Here's how the part is built. I have some questions about the finished solid (model axes, mm). Face numbers are marked on the shaded views. A direction names the side the tool comes from. Round coordinates to 2 decimals unless told otherwise and drop trailing zeros. Write each loop counter-clockwise with the first axis right and the second up, starting at its lowest first coordinate (ties: lowest second). Pieces come first, ordered by that corner, then holes. Notation, with made-up numbers: M 18,70.25 L 47,70.25 A34 ccw 47,105.25 Z; hole C 37.5,20 d11. An arc over 180 degrees is marked long. Use one line per item in the form item = value. Start each with the question number.
Q1. I want a section at D-D on x = -4.25. List the corners of the cut face in (y, z) for me, and give its area (3 significant figures).
Q2. I need wall thicknesses on line 1 along X through (y, z) = (-0.5, 10.75); line 2 along X through (y, z) = (3, 7.5); line 3 along Z through (x, y) = (-3.75, 10). Which ranges of each line are inside material? Lowest first, please. Write a range as from..to.
Q3. For the marked faces 1, 2 and 3, which set-ups out of +Z, -Z, +X, -X, +Y, -Y let a thin tool reach every point of the face, with its end or its side?
Q4. I want a section at B-B on z = 12.75. List the corners of the cut face in (x, y) for me.
Q5. I want a section at A-A on y = -1.5. List the corners of the cut face in (x, z) for me.
Q6. We'd pull the mould along Z, two halves only. Please class the marked faces 4, 5, 6 and 7: +Z half, -Z half, draft (parallel to the pull), parting line (faces both ways), or undercut.
Q7. I'm going to push flat-ended pins straight in: pin 1 Ø1.5 at (x, y) = (2, 10.5) entering from +Z; pin 2 Ø5.5 at (x, z) = (0, 7.5) entering from -Y; pin 3 Ø5.5 at (x, z) = (-2.5, 2.5) entering from +Y. Where does each tip first touch, or does it pass through?
Q8. I want a section at C-C on x = 0. List the corners of the cut face in (y, z) for me.
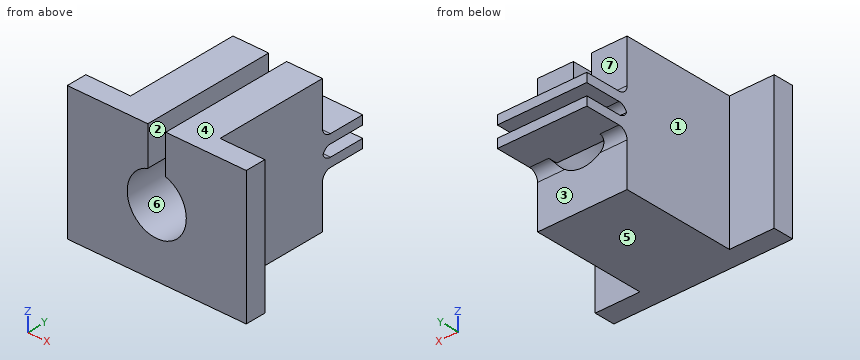
```python
from build123d import *

# Parameters (mm, degrees)
SKETCH1_W           = 10
SKETCH1_H           = 15
BOSS_EXTRUDE1_DEPTH = 15
SKETCH3_W           = 5
SKETCH3_H           = 2.3
BOSS_EXTRUDE2_DEPTH = 15
SKETCH4_R           = 3.3
CUT_EXTRUDE1_DEPTH  = 24.452078799
SKETCH6_W           = 2
SKETCH6_H           = 15
CUT_EXTRUDE2_DEPTH  = 8
SKETCH7_W           = 10
SKETCH7_H           = 1
BOSS_EXTRUDE3_DEPTH = 5
FILLET1_R           = 1


with BuildPart() as part:
    # Sketch1 → Boss-Extrude1 (new body)
    with BuildSketch(Plane.XY):
        Rectangle(SKETCH1_W, SKETCH1_H)
    extrude(amount=BOSS_EXTRUDE1_DEPTH)

    # Sketch3 → Boss-Extrude2 (add)
    with BuildSketch(Plane.XY.offset(15)):
        with Locations((-7.5, -6.35)):
            Rectangle(SKETCH3_W, SKETCH3_H)
        with Locations((7.5, -6.35)):
            Rectangle(SKETCH3_W, SKETCH3_H)
    extrude(amount=-BOSS_EXTRUDE2_DEPTH)

    # Sketch4 → Cut-Extrude1 (cut, through all)
    with BuildSketch(Plane.XZ.offset(7.5)):
        with Locations(Location((0, 7.5, 0), (0, 0, 270))):
            Circle(SKETCH4_R)
    extrude(amount=-CUT_EXTRUDE1_DEPTH, mode=Mode.SUBTRACT)

    # Sketch6 → Cut-Extrude2 (cut)
    with BuildSketch(Plane.XY.offset(15)):
        Rectangle(SKETCH6_W, SKETCH6_H)
    extrude(amount=-CUT_EXTRUDE2_DEPTH, mode=Mode.SUBTRACT)

    # Sketch7 → Boss-Extrude3 (add)
    with BuildSketch(Plane(origin=(0, 7.5, 0), x_dir=(1, 0, 0), z_dir=(0, 1, 0))):
        with Locations((0, -8.65)):
            Rectangle(SKETCH7_W, SKETCH7_H)
        with Locations((0, -6.35)):
            Rectangle(SKETCH7_W, SKETCH7_H)
    extrude(amount=BOSS_EXTRUDE3_DEPTH)

    # Fillet1
    # the kernel refuses this fillet: 1 mm, written as the material it adds along each edge
    with BuildSketch(Plane(origin=(5, 7.5, 5.85), x_dir=(0, 0, -1), z_dir=(-1, 0, 0))) as fillet1_piece_1_section:
        with BuildLine():
            CenterArc((FILLET1_R, -FILLET1_R), FILLET1_R, 90, 90)
            Line((0, -FILLET1_R), (0, 0))
            Line((0, 0), (FILLET1_R, 0))
        make_face()
    fillet1_piece_1 = extrude(amount=4.642116168, mode=Mode.PRIVATE)
    fillet1_piece_1 = fillet1_piece_1 - Plane(origin=(0, 7.716795794, 7.5), x_dir=(0, 0, -1), z_dir=(0, -1, 0)) * Cylinder(3.3, 14, mode=Mode.PRIVATE)
    add(fillet1_piece_1)
    with BuildSketch(Plane(origin=(0.735351604, 7.5, 6.85), x_dir=(0, 0, 1), z_dir=(1, 0, 0))) as fillet1_piece_2_section:
        with BuildLine():
            CenterArc((FILLET1_R, -FILLET1_R), FILLET1_R, 90, 90)
            Line((0, -FILLET1_R), (0, 0))
            Line((0, 0), (FILLET1_R, 0))
        make_face()
    fillet1_piece_2 = extrude(amount=4.264648396, mode=Mode.PRIVATE)
    fillet1_piece_2 = fillet1_piece_2 - Plane(origin=(0, 7.724716743, 7.5), x_dir=(0, 0, -1), z_dir=(0, -1, 0)) * Cylinder(3.3, 13, mode=Mode.PRIVATE)
    add(fillet1_piece_2)
    with BuildSketch(Plane(origin=(-0.357883832, 7.5, 5.85), x_dir=(0, 0, -1), z_dir=(-1, 0, 0))) as fillet1_piece_3_section:
        with BuildLine():
            CenterArc((FILLET1_R, -FILLET1_R), FILLET1_R, 90, 90)
            Line((0, -FILLET1_R), (0, 0))
            Line((0, 0), (FILLET1_R, 0))
        make_face()
    fillet1_piece_3 = extrude(amount=4.642116168, mode=Mode.PRIVATE)
    fillet1_piece_3 = fillet1_piece_3 - Plane(origin=(0, 7.716795859, 7.5), x_dir=(0, 0, -1), z_dir=(0, -1, 0)) * Cylinder(3.3, 14, mode=Mode.PRIVATE)
    add(fillet1_piece_3)
    with BuildSketch(Plane(origin=(-5, 7.5, 6.85), x_dir=(0, 0, 1), z_dir=(1, 0, 0))) as fillet1_piece_4_section:
        with BuildLine():
            CenterArc((FILLET1_R, -FILLET1_R), FILLET1_R, 90, 90)
            Line((0, -FILLET1_R), (0, 0))
            Line((0, 0), (FILLET1_R, 0))
        make_face()
    fillet1_piece_4 = extrude(amount=4.264648396, mode=Mode.PRIVATE)
    fillet1_piece_4 = fillet1_piece_4 - Plane(origin=(0, 7.724717828, 7.5), x_dir=(0, 0, -1), z_dir=(0, -1, 0)) * Cylinder(3.3, 13, mode=Mode.PRIVATE)
    add(fillet1_piece_4)
    with BuildSketch(Plane(origin=(-0.735351604, 7.5, 8.15), x_dir=(0, 0, -1), z_dir=(-1, 0, 0))) as fillet1_piece_5_section:
        with BuildLine():
            CenterArc((FILLET1_R, -FILLET1_R), FILLET1_R, 90, 90)
            Line((0, -FILLET1_R), (0, 0))
            Line((0, 0), (FILLET1_R, 0))
        make_face()
    fillet1_piece_5 = extrude(amount=4.264648396, mode=Mode.PRIVATE)
    fillet1_piece_5 = fillet1_piece_5 - Plane(origin=(0, 7.724716743, 7.5), x_dir=(0, 0, -1), z_dir=(0, -1, 0)) * Cylinder(3.3, 13, mode=Mode.PRIVATE)
    add(fillet1_piece_5)
    with BuildSketch(Plane(origin=(5, 7.5, 8.15), x_dir=(0, 0, -1), z_dir=(-1, 0, 0))) as fillet1_piece_6_section:
        with BuildLine():
            CenterArc((FILLET1_R, -FILLET1_R), FILLET1_R, 90, 90)
            Line((0, -FILLET1_R), (0, 0))
            Line((0, 0), (FILLET1_R, 0))
        make_face()
    fillet1_piece_6 = extrude(amount=4.264648396, mode=Mode.PRIVATE)
    fillet1_piece_6 = fillet1_piece_6 - Plane(origin=(0, 7.724717828, 7.5), x_dir=(0, 0, -1), z_dir=(0, -1, 0)) * Cylinder(3.3, 13, mode=Mode.PRIVATE)
    add(fillet1_piece_6)
    with BuildSketch(Plane(origin=(-5, 7.5, 9.15), x_dir=(0, 0, 1), z_dir=(1, 0, 0))) as fillet1_piece_7_section:
        with BuildLine():
            CenterArc((FILLET1_R, -FILLET1_R), FILLET1_R, 90, 90)
            Line((0, -FILLET1_R), (0, 0))
            Line((0, 0), (FILLET1_R, 0))
        make_face()
    fillet1_piece_7 = extrude(amount=4.642116168, mode=Mode.PRIVATE)
    fillet1_piece_7 = fillet1_piece_7 - Plane(origin=(0, 7.716795794, 7.5), x_dir=(0, 0, -1), z_dir=(0, -1, 0)) * Cylinder(3.3, 14, mode=Mode.PRIVATE)
    add(fillet1_piece_7)
    with BuildSketch(Plane(origin=(0.357883832, 7.5, 9.15), x_dir=(0, 0, 1), z_dir=(1, 0, 0))) as fillet1_piece_8_section:
        with BuildLine():
            CenterArc((FILLET1_R, -FILLET1_R), FILLET1_R, 90, 90)
            Line((0, -FILLET1_R), (0, 0))
            Line((0, 0), (FILLET1_R, 0))
        make_face()
    fillet1_piece_8 = extrude(amount=4.642116168, mode=Mode.PRIVATE)
    fillet1_piece_8 = fillet1_piece_8 - Plane(origin=(0, 7.716795859, 7.5), x_dir=(0, 0, -1), z_dir=(0, -1, 0)) * Cylinder(3.3, 14, mode=Mode.PRIVATE)
    add(fillet1_piece_8)


solid = part.part
```
Reported:
q1.outline = M -7.5,0 L 7.5,0 L 7.5,4.85 A1 cw 8.5,5.85 L 12.5,5.85 L 12.5,6.85 L 8.5,6.85 A1 cw 7.56,7.5 A1 cw 8.5,8.15 L 12.5,8.15 L 12.5,9.15 L 8.5,9.15 A1 cw 7.5,10.15 L 7.5,15 L -7.5,15 Z
q1.area = 236 mm^2
q2.line_1 = -5..-1, 1..5
q2.line_2 = -5..-3.3, 3.3..5
q2.line_3 = 5.85..6.85, 8.15..9.15
q3.face_1 = +Z, -Z, -X, +Y
q3.face_2 = +Z, +Y, -Y
q3.face_3 = -Z, +X, -X, +Y
q4.outline = M -10,-7.5 L -1,-7.5 L -1,7.5 L -5,7.5 L -5,-5.2 L -10,-5.2 Z; M 1,-7.5 L 10,-7.5 L 10,-5.2 L 5,-5.2 L 5,7.5 L 1,7.5 Z
q5.outline = M -5,0 L 5,0 L 5,15 L 1,15 L 1,10.64 A3.3 cw long -1,10.64 L -1,15 L -5,15 Z
q6.face_4 = +Z half
q6.face_5 = -Z half
q6.face_6 = undercut
q6.face_7 = draft
q7.pin_1 = 9.15
q7.pin_2 = 7.5
q7.pin_3 = 7.58
q8.outline = M -7.5,0 L 7.5,0 L 7.5,4.2 L -7.5,4.2 Z; M 7.5,5.85 L 12.5,5.85 L 12.5,6.85 L 7.5,6.85 Z; M 7.5,8.15 L 12.5,8.15 L 12.5,9.15 L 7.5,9.15 Z
